Here's how the part is built. I have some questions about the finished solid (model axes, mm). A direction names the side the tool comes from. Coordinates: 2 decimals unless noted, no trailing zeros. Loops run counter-clockwise (first coordinate to the right, second up) from the corner with the lowest first, then second, coordinate; pieces in that order, holes last. Notation, with made-up numbers: M -9,68.25 L 1,68.25 A16 cw 1,78.25 Z; hole C 56.5,12 d2. An arc over 180 degrees is marked long. Use one line per item in the form item = value. Start each with the question number.
(1) Imagine slicing it at A-A, the plane x = 0. Please give me the cut outline in (y, z), and give its area (3 significant figures).
(2) Imagine slicing it at D-D, the plane z = 4. Please give me the cut outline in (x, y).
(3) Imagine slicing it at C-C, the plane y = 0. Please give me the cut outline in (x, z).
(4) Thinking about a two-plate mould opening in Y: for faces 1 (the flat face through (0, -5.306, 3)), 2 (the flat face through (0, 0, 5.4)), 3 (the cylindrical face through (-2.21, -9.96, 5.2)), 4 (the flat face through (0, 5.306, 3)), which applies, +Y half, -Y half, draft (parallel to the pull), parting line (faces both ways), or undercut?
(5) Will these pins go through, and if not, where does the flat tip stop? P1, Ø1, axis at x = 3.5, y = -6, coming from the -Z side; P2, Ø1.1, axis at x = 0.5, z = 2.5, coming from the -Y side; P3, Ø1.9, axis at x = -0.5, z = 3.5, coming from the +Y side; P4, Ø0.8, axis at x = -0.5, y = 6, coming from the -Z side.
(6) Imagine slicing it at B-B, the plane z = 0.45. Please give me the cut outline in (x, y).
(7) Please list where these lines run through material, in increasing order: L1, parallel to Z at x = 3.5, y = -7.5; L2, parallel to Y at x = 1.75, z = 3.05; L3, parallel to X at y = -7.5, z = 1.1.
(8) On a 3-axis mill with a long thin cutter (end or side, diameter ignored), from which of +Z, -Z, +X, -X, +Y, -Y can I reach the whole of each face in a straight line? I mean faces 5 (the flat face through (0, 6, 0.5)), 6 (the flat face through (0, 7, 0)). Say none if no direction works.
```python
from build123d import *

# Parameters (mm, degrees)
F1_DEPTH = 5
F2_DEPTH = 1
F3_W     = 7.4393213727
F3_H     = 10.612742044
F4_DEPTH = 25
F5_R     = 10.2019510015
F6_DEPTH = 0.4


with BuildPart() as f1:
    # F0 (on Top) → F1 (new body)
    with BuildSketch(Plane.XY):
        with BuildLine():
            Line((-2, 6), (2, 6))
            ThreePointArc((2, 6), (0, 8), (-2, 6))
        make_face()
        with BuildLine():
            ThreePointArc((-2, 6), (0, 4), (2, 6))
            Line((2, 6), (-2, 6))
        make_face()
    extrude(amount=F1_DEPTH)


with BuildPart() as f1b:
    # F0 (on Top) → F1, piece 2 (new body)
    with BuildSketch(Plane.XY):
        with BuildLine():
            Line((-2, -6), (2, -6))
            ThreePointArc((2, -6), (0, -4), (-2, -6))
        make_face()
        with BuildLine():
            ThreePointArc((-2, -6), (0, -8), (2, -6))
            Line((2, -6), (-2, -6))
        make_face()
    extrude(amount=F1_DEPTH)


with BuildPart() as f2_tool:
    # F0 (on Top) → F2 (new body)
    with BuildSketch(Plane.XY):
        with BuildLine():
            ThreePointArc((-2, 6), (0, 4), (2, 6))
            Line((2, 6), (-2, 6))
        make_face()
        with BuildLine():
            Line((-2, -6), (2, -6))
            ThreePointArc((2, -6), (0, -4), (-2, -6))
        make_face()
    extrude(amount=F2_DEPTH)


with BuildPart() as f1_1:
    add(f1.part)

    # F2: cut by f2_tool
    add(f2_tool.part, mode=Mode.SUBTRACT)


with BuildPart() as f1b_1:
    add(f1b.part)

    # F2: cut by f2_tool
    add(f2_tool.part, mode=Mode.SUBTRACT)


with BuildPart() as f4_tool:
    # F3 (on face) → F4 (new body)
    with BuildSketch(Plane.XY):
        Rectangle(F3_W, F3_H)
    extrude(amount=F4_DEPTH)


with BuildPart() as f1_2:
    add(f1_1.part)

    # F4: cut by f4_tool
    add(f4_tool.part, mode=Mode.SUBTRACT)



with BuildPart() as f1b_2:
    add(f1b_1.part)

    # F4: cut by f4_tool
    add(f4_tool.part, mode=Mode.SUBTRACT)


with BuildPart() as f1_3:
    add(f1_2.part)

    add(f1b_2.part)  # F6 merges F1b
    # F5 (on face) → F6 (join)
    with BuildSketch(Plane.XY.offset(5)):
        Circle(F5_R)
    extrude(amount=F6_DEPTH)


solid = f1_3.part
```
Answer:
q1.outline = M -10.2,5 L -8,5 L -8,0 L -6,0 L -6,1 L -5.31,1 L -5.31,5 L 5.31,5 L 5.31,1 L 6,1 L 6,0 L 8,0 L 8,5 L 10.2,5 L 10.2,5.4 L -10.2,5.4 Z
q1.area = 33.7 mm²
q2.outline = M -1.88,-5.31 A2 ccw long 1.88,-5.31 Z; M -1.88,5.31 L 1.88,5.31 A2 ccw long Z
q3.outline = M -10.2,5 L 10.2,5 L 10.2,5.4 L -10.2,5.4 Z
q4.face_1 = undercut
q4.face_2 = draft
q4.face_3 = parting line
q4.face_4 = undercut
q5.P1 = 5
q5.P2 = -8
q5.P3 = 8
q5.P4 = 0
q6.outline = M -2,-6 A2 ccw 2,-6 Z; M -2,6 L 2,6 A2 ccw Z
q7.L1 = 5 to 5.4
q7.L2 = -6.97 to -5.31, 5.31 to 6.97
q7.L3 = -1.32 to 1.32
q8.face_5 = -Z, +X, -X
q8.face_6 = -Z, +X, -X, +Y, -Y
